```python
from build123d import *

# Parameters (mm, degrees)
CROQUIS4_R              = 1.267922183
SALIENTE_EXTRUIR3_DEPTH = 2.5
SALIENTE_EXTRUIR4_DEPTH = 2.5


with BuildPart() as part:
    # Croquis4 → Saliente-Extruir3 (new body)
    with BuildSketch(Plane.XY):
        with BuildLine():
            Line((30.406912218, -15.136800989), (30.406912218, 22.863199011))
            ThreePointArc((30.406912218, 22.863199011), (28.356659686, 27.812946479), (23.406912218, 29.863199011))
            Line((23.406912218, 29.863199011), (-29.593087782, 29.863199011))
            Line((-29.593087782, 29.863199011), (-29.593087782, -15.136800989))
            Line((-29.593087782, -15.136800989), (30.406912218, -15.136800989))
        make_face()
        with Locations((-20.564298519, 16.363199011)):
            Circle(CROQUIS4_R, mode=Mode.SUBTRACT)
    extrude(amount=SALIENTE_EXTRUIR3_DEPTH)

    # Croquis5 → Saliente-Extruir4 (add)
    with BuildSketch(Plane.XZ.offset(15.136800989)):
        with BuildLine():
            Line((30.406912218, 13.031466978), (30.406912218, -6.968533022))
            ThreePointArc((30.406912218, -6.968533022), (29.235339342, -9.796960146), (26.406912218, -10.968533022))
            Line((26.406912218, -10.968533022), (-45.593087782, -10.968533022))
            ThreePointArc((-45.593087782, -10.968533022), (-48.421514907, -9.796960146), (-49.593087782, -6.968533022))
            Line((-49.593087782, -6.968533022), (-49.593087782, 13.031466978))
            ThreePointArc((-49.593087782, 13.031466978), (-48.421514907, 15.859894103), (-45.593087782, 17.031466978))
            Line((-45.593087782, 17.031466978), (26.406912218, 17.031466978))
            ThreePointArc((26.406912218, 17.031466978), (29.235339342, 15.859894103), (30.406912218, 13.031466978))
        make_face()
    extrude(amount=SALIENTE_EXTRUIR4_DEPTH)


solid = part.part
```
The model under review builds one solid part; all positions refer to its coordinate system, in mm. A direction names the side the tool comes from. Coordinates: 2 decimals unless noted, no trailing zeros. Write each loop counter-clockwise with the first axis right and the second up, starting at its lowest first coordinate (ties: lowest second). Pieces come first, ordered by that corner, then holes. Notation, with made-up numbers: (14.25, 21) - (66.25, 21) arc R20 cw to (66.25, 31) - close; hole circle Ø7 at (9, -39). An arc over 180 degrees is marked (long way). Answer in a Markdown table with one row per item. Add a question column.
Q1. To check wall thickness, follow line 1 along Z through (x, y) = (-26.5, 24); line 2 along X through (y, z) = (15, 2.25); line 3 along Y through (x, z) = (25.5, 11.25). State the ranges of each line that lie inside material, in increasing order. Write a range as from..to.
Q2. Clearance check with flat-ended pins moving along their axes: pin 1 (12 mm diameter, centred on x = 1.5, y = 1, fed in from +Z); pin 2 (5 mm diameter, centred on x = -3.5, y = 23.5, fed in from -Z); pin 3 (5 mm diameter, centred on x = -37, y = -12, fed in from -Z); pin 4 (1.2 mm diameter, centred on y = 18, z = 1.5, fed in from -X). State where each tip first meets the part, or that it passes through.
Q3. Draft analysis for pull direction X (two halves, no side actions). For faces 1 (the face through (29.266, -16.369, -9.766)), 2 (the face through (-9, -17.637, 3)), 3 (the face through (-19.98, 15.24, 1.23)), state which applies: +X half, -X half, draft (parallel to the pull), parting line (faces both ways), or undercut.
Q4. Consider section A-A on x = -11. Give the boundary of the cut face in (y, z), then the cut area to 4 significant figures.
Q5. Consider section B-B on z = 10.75. Give the boundary of the cut face in (x, y).
Q6. Consider section C-C on y = 22. Give the boundary of the cut face in (x, z).
Q7. For faces 4 (the face through (0, 8, 2.5)), 5 (the face through (0, 8, 0)), 6 (the face through (28.41, 27.76, 1.23)), 7 (the face through (-29.593, 8, 1)), list the 3-axis set-ups (+Z, -Z, +X, -X, +Y, -Y) from which the entire face can be reached by the end or side of a thin tool; tool diameter is ignored.
Answers below:
| question | item | result |
|---|---|---|
| 1 | line 1 | 0..2.5 |
| 1 | line 2 | -29.59..30.41 |
| 1 | line 3 | -17.64..-15.14 |
| 2 | pin 1 | z = 2.5 |
| 2 | pin 2 | z = 0 |
| 2 | pin 3 | through |
| 2 | pin 4 | x = -29.59 |
| 3 | face 1 | +X half |
| 3 | face 2 | draft |
| 3 | face 3 | undercut |
| 4 | outline | (-17.64, -10.97) - (-15.14, -10.97) - (-15.14, 0) - (29.86, 0) - (29.86, 2.5) - (-15.14, 2.5) - (-15.14, 17.03) - (-17.64, 17.03) - close |
| 4 | area | 182.5 mm² |
| 5 | outline | (-49.59, -17.64) - (30.41, -17.64) - (30.41, -15.14) - (-49.59, -15.14) - close |
| 6 | outline | (-29.59, 0) - (30.41, 0) - (30.41, 2.5) - (-29.59, 2.5) - close |
| 7 | face 4 | +Z, +X, -X, +Y |
| 7 | face 5 | -Z, +X, -X, +Y |
| 7 | face 6 | +Z, -Z, +X, +Y |
| 7 | face 7 | +Z, -Z, -X, +Y |
